Verification items for the finished model (mm, model axes). A direction names the side the tool comes from. Give positions to 0.01 mm unless a question says otherwise; leave off trailing zeros. Write each loop counter-clockwise with the first axis right and the second up, starting at its lowest first coordinate (ties: lowest second). Pieces come first, ordered by that corner, then holes.
Autodesk Inventor part; units mm, degrees
ref_plane "YZ Plane" through (0, 0, 0) normal (1, 0, 0) x (0, 1, 0)
ref_plane "XZ Plane" through (0, 0, 0) normal (0, 1, 0) x (-1, 0, 0)
ref_plane "XY Plane" through (0, 0, 0) normal (0, 0, 1) x (1, 0, 0)
sketch "Sketch1" plane through (0, 0, 0) normal (0, 1, 0) x (-1, 0, 0)
  circle A0 centre (0, 0) radius 25.9
  circle A1 centre (0, 0) radius 25
  circle A2 centre (0, 0) radius 26.8
  dimension "d0" = 51.8
  dimension "d1" = 50
  dimension "d2" = 53.6
extrude "Extrusion1" add sketch "Sketch1" along normal mid plane 100 contours A0
extrude "Extrusion2" add sketch "Sketch1" along normal blind 45 and the other way blind 55 contours A2
properties part number "extraTube" material "ABS Plastic"
Item 1: Release check for a two-part mould opening along X. For faces 1 (the face through (-23.846, -0.7, -7.509)), 2 (the face through (5.615, 47.465, 25.284)), 3 (the face through (14, 45, 22)) record: released by +X, released by -X, zero draft, split by the parting line, or undercut.
Answer key:
face 1: undercut
face 2: split by the parting line
face 3: zero draft
Item 2: Sectioned sample at C-C on y = -36. Record the cut outline in (x, z).
Answer key:
outline: circle Ø53.6 at (0, 0); hole circle Ø50 at (0, 0)
Item 3: Sectioned sample at A-A on z = 0. Record the cut outline in (x, y), then the cut area to 3 significant figures.
Answer key:
outline: (-26.8, -55) - (-25.9, -55) - (-25.9, -50) - (-25, -50) - (-25, 50) - (-25.9, 50) - (-25.9, 45) - (-26.8, 45) - close; (25, -50) - (25.9, -50) - (25.9, -55) - (26.8, -55) - (26.8, 45) - (25.9, 45) - (25.9, 50) - (25, 50) - close
area: 360 mm2
Item 4: Set-up check for faces 4 (the face through (5.615, -52.465, -25.284)), 5 (the face through (21, 50, 14)): record each of +Z, -Z, +X, -X, +Y, -Y from which the full face is reachable in a straight line by a thin tool's end or side.
Answer key:
face 4: -Y
face 5: +Z, -Z, +X, -X, +Y
Item 5: Scan lines: line 1 along Z through (x, y) = (0, 18); line 2 along Z through (x, y) = (-21.5, 30); line 3 along X through (y, z) = (38.5, -1). Record each from-to range of solid material in increasing order.
Answer key:
line 1: z = -26.8 to -25, 25 to 26.8
line 2: z = -16 to -12.76, 12.76 to 16
line 3: x = -26.78 to -24.98, 24.98 to 26.78
Item 6: Depth check by flat-ended pin: pin 1 (1 mm diameter, centred on x = 6, y = 24, fed in from +Z); pin 2 (1 mm diameter, centred on y = 38.5, z = 10, fed in from +X); pin 3 (6 mm diameter, centred on x = 9, y = 2.5, fed in from -Z). Enter the tip coordinate at first touch or a pass-through.
Answer key:
pin 1: stops at z = 26.23
pin 2: stops at x = 25.06
pin 3: stops at z = -26.12
Item 7: Sectioned sample at B-B on x = 0. Record the cut outline in (y, z).
Answer key:
outline: (-55, -26.8) - (45, -26.8) - (45, -25.9) - (50, -25.9) - (50, -25) - (-50, -25) - (-50, -25.9) - (-55, -25.9) - close; (-55, 25.9) - (-50, 25.9) - (-50, 25) - (50, 25) - (50, 25.9) - (45, 25.9) - (45, 26.8) - (-55, 26.8) - close
